Can you work these out from the model? Positions are in its coordinate system, mm. A direction names the side the tool comes from. Give positions to 0.01 mm unless a question says otherwise; leave off trailing zeros. Write each loop counter-clockwise with the first axis right and the second up, starting at its lowest first coordinate (ties: lowest second). Pieces come first, ordered by that corner, then holes.
```python
from build123d import *

# Parameters (mm, degrees)
SKETCH1_R           = 18.25
SKETCH1_R_2         = 13.25
BOSS_EXTRUDE1_DEPTH = 18
SKETCH2_R           = 26.25
SKETCH2_R_2         = 13.25
FLANGE_DEPTH        = 5
CUT_EXTRUDE1_REACH  = 43.257
SKETCH4_R           = 1.5
CIRPATTERN1_COUNT   = 8
SKETCH6_R           = 18.25
SKETCH6_R_2         = 3.5
TOP_DEPTH           = 5
SKETCH7_R           = 26.25
SKETCH7_R_2         = 19.25
SKETCH7_R_3         = 1.5
BOSS_EXTRUDE5_DEPTH = 10
FILLET1_R           = 2


with BuildPart() as part:
    # Sketch1 → Boss-Extrude1 (new body)
    with BuildSketch(Plane(origin=(0, 0, 0), x_dir=(1, 0, 0), z_dir=(0, 1, 0))):
        with Locations(Location((0, 0, 0), (0, 0, 270))):
            Circle(SKETCH1_R)
        with Locations(Location((0, 0, 0), (0, 0, 270))):
            Circle(SKETCH1_R_2, mode=Mode.SUBTRACT)
    extrude(amount=BOSS_EXTRUDE1_DEPTH)

    # Sketch2 → flange (add)
    with BuildSketch(Plane.XZ):
        with Locations(Location((0, 0, 0), (0, 0, 270))):
            Circle(SKETCH2_R)
        with Locations(Location((0, 0, 0), (0, 0, 270))):
            Circle(SKETCH2_R_2, mode=Mode.SUBTRACT)
    extrude(amount=FLANGE_DEPTH)

    # Sketch4 → Cut-Extrude1 (cut, up to next)
    with BuildSketch(Plane(origin=(0, 0, 0), x_dir=(1, 0, 0), z_dir=(0, 1, 0)), mode=Mode.PRIVATE) as cut_extrude1_sk1:
        with Locations(Location((0, -22.25, 0), (0, 0, 270))):
            Circle(SKETCH4_R)
    cut_extrude1_tool1 = extrude(cut_extrude1_sk1.sketch, amount=-CUT_EXTRUDE1_REACH, mode=Mode.PRIVATE) & part.part
    cut_extrude1 = cut_extrude1_tool1.solids().sort_by_distance((0, 0, 22.25))[0]
    add(cut_extrude1, mode=Mode.SUBTRACT)

    # CirPattern1: Cut-Extrude1 ×8 about axis
    cirpattern1_axis = Axis((0, 0, 0), (0, 1, 0))
    for i in range(1, CIRPATTERN1_COUNT):
        add(cut_extrude1.rotate(cirpattern1_axis, i * 360 / CIRPATTERN1_COUNT), mode=Mode.SUBTRACT)

    # Sketch6 → top (add)
    with BuildSketch(Plane(origin=(0, 18, 0), x_dir=(1, 0, 0), z_dir=(0, 1, 0))):
        with Locations(Location((0, 0, 0), (0, 0, 270))):
            Circle(SKETCH6_R)
        with Locations(Location((0, 0, 0), (0, 0, 270))):
            Circle(SKETCH6_R_2, mode=Mode.SUBTRACT)
    extrude(amount=TOP_DEPTH)

    # Sketch7 → Boss-Extrude5 (add)
    with BuildSketch(Plane.XZ.offset(5)):
        with Locations(Location((0, 0, 0), (0, 0, 270))):
            Circle(SKETCH7_R)
        with Locations(Location((0, 0, 0), (0, 0, 270))):
            Circle(SKETCH7_R_2, mode=Mode.SUBTRACT)
        with Locations(Location((-15.733125881, -15.733125881, 0), (0, 0, 225))):
            Circle(SKETCH7_R_3, mode=Mode.SUBTRACT)
        with Locations(Location((15.733125881, -15.733125881, 0), (0, 0, 315))):
            Circle(SKETCH7_R_3, mode=Mode.SUBTRACT)
        with Locations(Location((15.733125881, 15.733125881, 0), (0, 0, 45))):
            Circle(SKETCH7_R_3, mode=Mode.SUBTRACT)
        with Locations(Location((0, 22.25, 0), (0, 0, 90))):
            Circle(SKETCH7_R_3, mode=Mode.SUBTRACT)
        with Locations(Location((-15.733125881, 15.733125881, 0), (0, 0, 135))):
            Circle(SKETCH7_R_3, mode=Mode.SUBTRACT)
        with Locations((22.25, 0)):
            Circle(SKETCH7_R_3, mode=Mode.SUBTRACT)
        with Locations(Location((0, -22.25, 0), (0, 0, 270))):
            Circle(SKETCH7_R_3, mode=Mode.SUBTRACT)
        with Locations(Location((-22.25, 0, 0), (0, 0, 180))):
            Circle(SKETCH7_R_3, mode=Mode.SUBTRACT)
    extrude(amount=BOSS_EXTRUDE5_DEPTH)

    # Fillet1
    fillet1_edges = [part.edges().sort_by_distance(p)[0] for p in [
        (0, 23, -18.25),
    ]]
    fillet(fillet1_edges, radius=FILLET1_R)


solid = part.part
```
1) Suppose I cut it at C-C on y = 10. Write out the boundary of the cut face in (x, z), plus the area to 3 significant figures.
Values follow:
outline: circle Ø36.5 at (0, 0); hole circle Ø26.5 at (0, 0)
area: 495 mm2
2) Suppose I cut it at D-D on x = 22.25. Write out the boundary of the cut face in (y, z).
Values follow:
outline: (-15, -13.93) - (0, -13.93) - (0, -1.5) - (-15, -1.5) - close; (-15, 1.5) - (0, 1.5) - (0, 13.93) - (-15, 13.93) - close
3) Please list where these lines run through material, in increasing order: L1, parallel to X at y = 11, z = 0; L2, parallel to X at y = -11, z = 0; L3, parallel to X at y = -4, z = 0.
Values follow:
L1: x = -18.25 to -13.25, 13.25 to 18.25
L2: x = -26.25 to -23.75, -20.75 to -19.25, 19.25 to 20.75, 23.75 to 26.25
L3: x = -26.25 to -23.75, -20.75 to -13.25, 13.25 to 20.75, 23.75 to 26.25
4) For pin 1 Ø5 at (x, z) = (0, 22.25) entering from +Y; pin 2 Ø1.5 at (x, z) = (5, -6.5) entering from -Y; pin 3 Ø1.5 at (y, z) = (-1.5, -13.5) entering from +X, each with a flat end and sliding along its axis, tell me the tip position at first contact or that it passes through.
Values follow:
pin 1: stops at y = 0
pin 2: stops at y = 18
pin 3: stops at x = 22.95
5) For faces 1 (the face through (16, -15, 12)), 2 (the face through (-17.816, 10.353, -3.956)), 3 (the face through (-13, -5, 5)), which set-ups out of +Z, -Z, +X, -X, +Y, -Y let a thin tool reach every point of the face, with its end or its side?
Values follow:
face 1: +Z, -Z, +X, -X, -Y
face 2: +Y
face 3: -Y
6) Suppose I cut it at A-A on z = 0. State how many separate pieces and enclosed holes the cut face has, plus the area to 3 significant figures.
Values follow:
separate pieces: 4
enclosed holes: 0
area: 506 mm2
